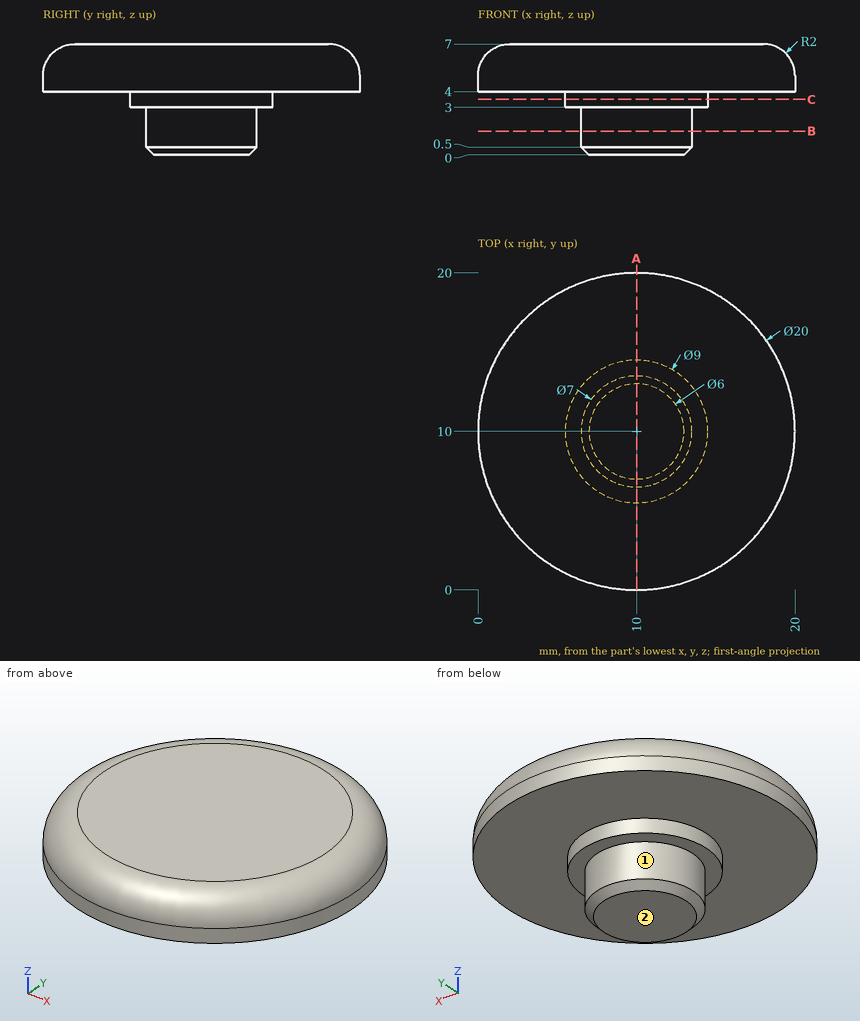
The drawing under review shows one solid part. Ordinate dimensions are in mm from its lowest x, y, z. A direction names the side the tool comes from. Round coordinates to 2 decimals unless told otherwise and drop trailing zeros. Write each loop counter-clockwise with the first axis right and the second up, starting at its lowest first coordinate (ties: lowest second). Pieces come first, ordered by that corner, then holes.
(1) We need section B-B on z = 1.5. Give the boundary of the cut face in (x, y).
(2) Machinability: for the marked faces 1 and 2, which of the approach directions +Z, -Z, +X, -X, +Y, -Y give a long, thin tool a straight path to every point of the face, cutting with its end or side? Answer none if there is none.
(3) Insertion check: pin 1 (2 mm diameter, centred on x = 16.5, z = 3.5, fed in from +Y); pin 2 (2 mm diameter, centred on x = 11, z = 1, fed in from -Y); pin 3 (1 mm diameter, centred on x = 4.5, y = 5.5, fed in from -Z). Each pin has a flat end and moves straight along its axis. Give the tip position at first contact, or say it passes through.
(4) We need section C-C on z = 3.5. Give the boundary of the cut face in (x, y), and give its area (3 significant figures).
(5) We need section A-A on x = 10. Give the boundary of the cut face in (y, z).
(6) Wall thickness on L1, parallel to Z at x = 5.75, y = 9.25; L2, parallel to Z at x = 2.75, y = 6.75; L3, parallel to X at y = 9, z = 4.25: over which ranges is each line inside the solid? List them lowest first.
Findings below:
1. outline: circle Ø7 at (10, 10)
2. face 1: -Z
2. face 2: -Z, +X, -X, +Y, -Y
3. pin 1: stops at y = 18.26
3. pin 2: stops at y = 6.5
3. pin 3: stops at z = 4
4. outline: circle Ø9 at (10, 10)
4. area: 63.6 mm2
5. outline: (0, 4) - (5.5, 4) - (5.5, 3) - (6.5, 3) - (6.5, 0.5) - (7, 0) - (13, 0) - (13.5, 0.5) - (13.5, 3) - (14.5, 3) - (14.5, 4) - (20, 4) - (20, 5) arc R2 ccw to (18, 7) - (2, 7) arc R2 ccw to (0, 5) - close
6. L1: z = 3 to 7
6. L2: z = 4 to 7
6. L3: x = 0.05 to 19.95
